Input: dimensioned drawing with shaded views. Units: mm. Origin: part minimum x, y, z. A direction names the side the tool comes from. Round coordinates to 2 decimals unless told otherwise and drop trailing zeros. Loops run counter-clockwise (first coordinate to the right, second up) from the corner with the lowest first, then second, coordinate; pieces in that order, holes last. Notation, with made-up numbers: (32.25, 73) - (49.25, 73) arc R27 ccw to (49.25, 103) - close; hole circle Ø1 at (38, 82). An arc over 180 degrees is marked (long way). Answer as a JSON object with one key per item and string values. Group by question number.
Item 1: Section A-A (x = 3.87). Return the cut outline in (y, z).
Item 2: Reachability of the marked faces 4 and 5 from +Z, -Z, +X, -X, +Y, -Y: full face, straight path, thin tool, end or side. Return the list, or none.
Item 3: First-contact query: pin 1 (3 mm diameter, centred on x = 27, y = 10.5, fed in from -Z). Flat tip, straight axial feed; report the tip coordinate or a pass-through.
Item 4: Section C-C (z = 0.9). Count the separate pieces of the cut face and the enclosed holes in it, plus the area to 3 significant figures.
Item 5: Draft query along X for the marked faces 1, 2 and 3. Return one class per face: released by +X, released by -X, zero draft, split by the parting line, or undercut.
Item 6: Line query: line 1 (X direction, y = 19.75, z = 2.8); line 2 (Y direction, x = 28, z = 2.05); line 3 (X direction, y = 17.5, z = 0.7). Output: solid intervals per line, ascending.
Item 7: Section D-D (x = 22.5). Return the cut outline in (y, z), plus the area to 3 significant figures.
Item 8: Section B-B (y = 12.5). Return the cut outline in (x, z).
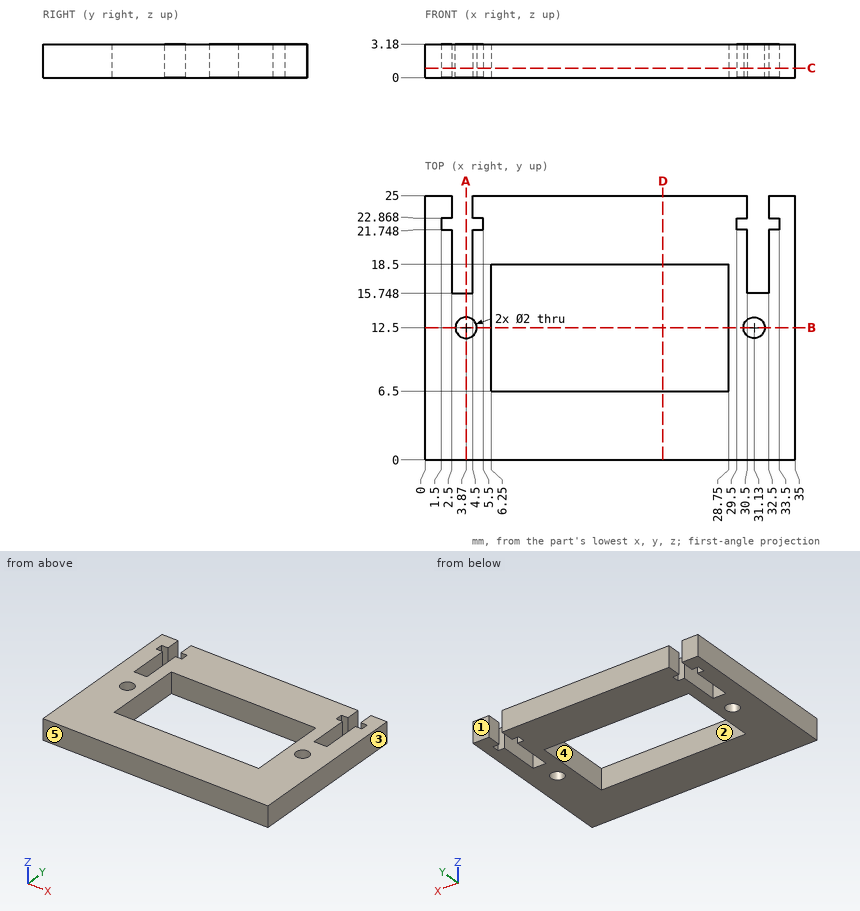
Values:
{
 "1": {"outline": "(0, 0) - (11.5, 0) - (11.5, 3.18) - (0, 3.18) - close; (13.5, 0) - (15.75, 0) - (15.75, 3.18) - (13.5, 3.18) - close"},
 "2": {"face 4": "+Z, -Z", "face 5": "+Z, -Z, +X, -X, -Y"},
 "3": {"pin 1": "passes through"},
 "4": {"separate pieces": "1", "enclosed holes": "3", "area": "557 mm^2"},
 "5": {"face 1": "zero draft", "face 2": "undercut", "face 3": "released by +X"},
 "6": {"line 1": "x = 0 to 2.5, 4.5 to 30.5, 32.5 to 35", "line 2": "y = 0 to 6.5, 18.5 to 25", "line 3": "x = 0 to 2.5, 4.5 to 6.25, 28.75 to 30.5, 32.5 to 35"},
 "7": {"outline": "(0, 0) - (6.5, 0) - (6.5, 3.18) - (0, 3.18) - close; (18.5, 0) - (25, 0) - (25, 3.18) - (18.5, 3.18) - close", "area": "41.3 mm^2"},
 "8": {"outline": "(0, 0) - (2.87, 0) - (2.87, 3.18) - (0, 3.18) - close; (4.87, 0) - (6.25, 0) - (6.25, 3.18) - (4.87, 3.18) - close; (28.75, 0) - (30.13, 0) - (30.13, 3.18) - (28.75, 3.18) - close; (32.13, 0) - (35, 0) - (35, 3.18) - (32.13, 3.18) - close"}
}
